Can you work these out from the model? Positions are in its coordinate system, mm. A direction names the side the tool comes from. Coordinates: 2 decimals unless noted, no trailing zeros. Order: outer loops, then holes, each group sorted by start corner. A loop starts at its lowest first (then second) coordinate and runs counter-clockwise, first axis right, second up. Notation, with made-up numbers: (-16, -29.5) -> (-5, -29.5) arc R30 cw to (-5, -7.5) -> close; hole circle Ø1 at (76, -18). An arc over 180 degrees is marked (long way). Write item = value, one per line.
```python
from build123d import *

# Parameters (mm, degrees)
CROQUIS1_R              = 1.5
SALIENTE_EXTRUIR1_DEPTH = 10
SALIENTE_EXTRUIR2_DEPTH = 15
SALIENTE_EXTRUIR3_DEPTH = 13
SALIENTE_EXTRUIR7_DEPTH = 5
REDONDEO2_R             = 10
SALIENTE_EXTRUIR8_DEPTH = 10


with BuildPart() as part:
    # Croquis1 → Saliente-Extruir1 (new body)
    with BuildSketch(Plane(origin=(0, 0, 0), x_dir=(1, 0, 0), z_dir=(0, 1, 0))):
        Polygon((-192.31475004, 37.351943635), (-153.149960772, 37.351943635), (-153.149960772, 29.769862991), (-126.147833027, 29.769862991), (-126.147833027, -29.769862991), (-153.149960772, -29.769862991), (-153.149960772, -9.1952793), (-192.31475004, -9.1952793), align=None)
        with Locations(Location((-137.631197841, -26.344824576, 0), (0, 0, 90))):
            Circle(CROQUIS1_R, mode=Mode.SUBTRACT)
    extrude(amount=SALIENTE_EXTRUIR1_DEPTH)

    # Croquis3 → Saliente-Extruir2 (add)
    with BuildSketch(Plane.XY.offset(9.1952793)):
        Polygon((-189.195504205, 0), (-201.604805992, 12.545329197), (-220.943628409, 69.680078214), (-231.495067756, 78.724169083), (-209.43357333, 78.724169083), (-189.195504205, 18.932679451), (-166.427858451, 10), (-166.427858451, 0), align=None)
    extrude(amount=-SALIENTE_EXTRUIR2_DEPTH)

    # Croquis8 → Saliente-Extruir3 (add)
    with BuildSketch(Plane(origin=(-163.998418841, -55.509761627, 0), x_dir=(0, 0, -1), z_dir=(0.9472114013741786, 0.3206096709501519, 0))):
        Polygon((5.8047207, 107.105877542), (5.8047207, 102.023441322), (17.229529669, 102.023441322), (17.229529669, 62.195551935), (21.649352835, 62.195551935), (21.649352835, 101.235469829), (41.412588148, 92.240137187), (41.412588148, 97.139259402), (18.703552524, 107.105877542), align=None)
    extrude(amount=-SALIENTE_EXTRUIR3_DEPTH)

    # Croquis10 → Saliente-Extruir7 (add)
    with BuildSketch(Plane(origin=(0, 78.724169083, 0), x_dir=(1, 0, 0), z_dir=(0, 1, 0))):
        with BuildLine():
            Line((-249.918671642, 64.972502389), (-235.980528396, 60.431124344))
            Line((-235.980528396, 60.431124344), (-233.719997047, 58.216185839))
            Line((-233.719997047, 58.216185839), (-209.380524185, 46.740483345))
            ThreePointArc((-209.380524185, 46.740483345), (-207.290181053, 44.895496777), (-206.512830069, 42.217954006))
            Line((-206.512830069, 42.217954006), (-206.512830069, 39.966009421))
            ThreePointArc((-206.512830069, 39.966009421), (-207.977296163, 36.430475515), (-211.512830069, 34.966009421))
            Line((-211.512830069, 34.966009421), (-212.273678507, 34.966009421))
            Line((-212.273678507, 34.966009421), (-212.273678507, 7.849044618))
            Line((-212.273678507, 7.849044618), (-211.512568985, 7.30119364))
            ThreePointArc((-211.512568985, 7.30119364), (-209.983572109, 5.522948339), (-209.43357333, 3.243148098))
            Line((-209.43357333, 3.243148098), (-209.43357333, -4.1952793))
            ThreePointArc((-209.43357333, -4.1952793), (-210.898039424, -7.730813206), (-214.43357333, -9.1952793))
            Line((-214.43357333, -9.1952793), (-231.495067756, -9.1952793))
            Line((-231.495067756, -9.1952793), (-233.719997047, -7.977642104))
            Line((-233.719997047, -7.977642104), (-235.980528396, -1.039745845))
            Line((-235.980528396, -1.039745845), (-249.918671642, -5.581123891))
            Line((-249.918671642, -5.581123891), (-264.188355718, 9.695689249))
            Line((-264.188355718, 9.695689249), (-249.918671642, 24.972502389))
            Line((-249.918671642, 24.972502389), (-235.980528396, 20.431124344))
            Line((-235.980528396, 20.431124344), (-222.964320543, 13.307743434))
            Line((-222.964320543, 13.307743434), (-218.531551458, 21.40752702))
            Line((-218.531551458, 21.40752702), (-218.531551458, 29.623801484))
            Line((-218.531551458, 29.623801484), (-235.980528396, 38.960254155))
            Line((-235.980528396, 38.960254155), (-249.918671642, 34.418876109))
            Line((-249.918671642, 34.418876109), (-264.188355718, 49.695689249))
            Line((-264.188355718, 49.695689249), (-249.918671642, 64.972502389))
        make_face()
    extrude(amount=SALIENTE_EXTRUIR7_DEPTH)

    # Redondeo2
    # the kernel refuses this fillet: 10 mm, written as the material it takes off along each edge
    with BuildSketch(Plane(origin=(-196.252662499, -0.765351442, 3.059587863), x_dir=(0.947211401374178, 0.3206096709501537, 0), z_dir=(0, 0, -1))) as redondeo2_piece_1:
        with BuildLine():
            CenterArc((10, -8.115647013), REDONDEO2_R, 125.75091012, 54.24908988)
            Line((0, -8.115647013), (-0.2, -8.115647013))
            Line((-0.2, -8.115647013), (-0.2, 0))
            Line((-0.2, 0), (0, 0.2))
            ThreePointArc((0, 0.2), (2.078687215, 0.2), (4.040521918, 0.16231294))
            Line((4.040521918, 0.16231294), (4.157374429, 0))
        make_face()
    extrude(amount=44.99805823, mode=Mode.SUBTRACT)

    # Croquis13 → Saliente-Extruir8 (add)
    with BuildSketch(Plane(origin=(0, 0, -37.351943635), x_dir=(-1, 0, 0), z_dir=(0, 0, -1))):
        with BuildLine():
            Line((192.31475004, 0), (201.604805992, 12.545329197))
            Line((201.604805992, 12.545329197), (220.943628409, 69.680078214))
            Line((220.943628409, 69.680078214), (227.212441383, 78.145508653))
            Line((227.212441383, 78.145508653), (211.22386426, 78.145508653))
            Line((211.22386426, 78.145508653), (184.515278381, 10))
            Line((184.515278381, 10), (177.732355406, 10))
            ThreePointArc((177.732355406, 10), (174.1968215, 8.535533906), (172.732355406, 5))
            Line((172.732355406, 5), (172.732355406, 0))
            Line((172.732355406, 0), (182.732355406, 0))
            Line((182.732355406, 0), (192.31475004, 0))
        make_face()
    extrude(amount=SALIENTE_EXTRUIR8_DEPTH)


solid = part.part
```
Item 1: I want a section at B-B, the plane z = -11.5. Please give me the cut outline in (x, y), plus the area to 3 significant figures.
A:
outline = (-262.5, 78.72) -> (-212.27, 78.72) -> (-212.27, 83.72) -> (-262.5, 83.72) -> close; (-210.65, 41.77) -> (-209.02, 36.96) -> (-196.71, 41.13) -> (-198.34, 45.94) -> close; (-192.31, 0) -> (-126.15, 0) -> (-126.15, 10) -> (-192.31, 10) -> close
area = 979 mm2
Item 2: I want a section at D-D, the plane z = 17.5. Please give me the cut outline in (x, y), plus the area to 3 significant figures.
A:
outline = (-153.15, 0) -> (-126.15, 0) -> (-126.15, 10) -> (-153.15, 10) -> close
area = 270 mm2
Item 3: If we mould it in two halves opening along Y, with no side actions, what happens to faces 6 (the flat face through (-219, 78.146, -42)), 7 (the flat face through (-151, 10, -9)), 8 (the flat face through (-257, 81, -42))? For each: pulls with the +Y half, pulls with the -Y half, needs draft (parallel to the pull), parting line crosses it, or undercut.
A:
face_6 = undercut
face_7 = pulls with the +Y half
face_8 = needs draft
Item 4: I want a section at C-C, the plane y = 59. Please give me the cut outline in (x, z).
A:
outline = (-217.33, -47.35) -> (-203.72, -47.35) -> (-203.72, -37.35) -> (-217.33, -37.35) -> close; (-217.33, -5.8) -> (-202.76, -5.8) -> (-202.76, 9.2) -> (-217.33, 9.2) -> close
Item 5: I'm going to push flat-ended pins straight in: P1, Ø3, axis at y = 3, z = -6, coming from the -X side; P2, Ø3, axis at y = 41, z = -1, coming from the +X side; P3, Ø4, axis at x = -191.5, y = 29.5, coming from the +Z side. Where does each tip first touch, or does it pass through?
A:
P1 = -193.63
P2 = -196.16
P3 = 9.2
Item 6: If I drill on probe 1 along Y at (x, z) = (-216, -26); probe 2 along X at (y, z) = (38, -40.5); probe 3 along Y at (x, z) = (-203.5, -13.5), over which ranges is the centre line in solid material (lowest first)?
A:
probe_1 = 78.72 to 83.72
probe_2 = -210.22 to -195.49
probe_3 = 38.83 to 44.19
Item 7: I want a section at A-A, the plane y = 24.5. Please give me the cut outline in (x, z).
A:
outline = (-205.65, -47.35) -> (-190.2, -47.35) -> (-190.2, -37.35) -> (-205.65, -37.35) -> close; (-205.65, -5.8) -> (-191.08, -5.8) -> (-191.08, 9.2) -> (-205.65, 9.2) -> close; (-204.8, -21.65) -> (-191.08, -21.65) -> (-191.08, -17.23) -> (-204.8, -17.23) -> close
Item 8: For faces 1 (the flat face through (-242.85, 81.19, 3.28)), 2 (the flat face through (-200, 36, -47.352)), 3 (the cylindrical face through (-207.31, 81.19, -44.93)), 4 (the flat face through (-243.047, 81.189, -22.734)), 5 (the cylindrical face through (-209.999, 81.189, -5.552)), which set-ups out of +Z, -Z, +X, -X, +Y, -Y let a thin tool reach every point of the face, with its end or its side?
A:
face_1 = +Z, +Y, -Y
face_2 = -Z, +X, -X, -Y
face_3 = -Z, +X, +Y
face_4 = +Y, -Y
face_5 = +X, +Y
